from build123d import *

# Parameters (mm, degrees)
BOSS_EXTRUDE1_DEPTH = 5
SKETCH8_R           = 3.5
BOSS_EXTRUDE5_DEPTH = 1.5
SKETCH10_R          = 8
BOSS_EXTRUDE7_DEPTH = 5.75
SKETCH15_R          = 2.8
CUT_EXTRUDE7_DEPTH  = 10
NUT_CUT_START       = -1.5
SKETCH6_W           = 8.4
SKETCH6_H           = 8.4
NUT_CUT_DEPTH       = 46.182751545
SKETCH16_W          = 12
SKETCH16_H          = 3
CUT_EXTRUDE8_DEPTH  = 23
SKETCH17_R          = 2.35
CUT_EXTRUDE9_DEPTH  = 28
CUT_EXTRUDE10_START = 1.5
SKETCH19_R          = 6.25
CUT_EXTRUDE10_DEPTH = 46.182751545
CUT_EXTRUDE11_START = -8
CUT_EXTRUDE11_DEPTH = 3.8
LPATTERN1_COUNT     = 2
LPATTERN1_PITCH     = 10
SKETCH22_R          = 3.051848234
BOSS_EXTRUDE8_DEPTH = 0.65
SKETCH23_R          = 3.919040969
BOSS_EXTRUDE9_DEPTH = 0.65


with BuildPart() as part:
    # Sketch1 → Boss-Extrude1 (new body)
    with BuildSketch(Plane.XY):
        with BuildLine():
            Line((-40.155138696, -0.836255417), (-17.155138696, -0.836255417))
            Line((-17.155138696, -0.836255417), (-5.68921993, -10.190248634))
            ThreePointArc((-5.68921993, -10.190248634), (6.973720426, -8.905748138), (5.68921993, 3.757192218))
            Line((5.68921993, 3.757192218), (-10.744236538, 17.163744583))
            Line((-10.744236538, 17.163744583), (-40.155138696, 17.163744583))
            Line((-40.155138696, 17.163744583), (-40.155138696, -0.836255417))
        make_face()
    extrude(amount=BOSS_EXTRUDE1_DEPTH)

    # Sketch8 → Boss-Extrude5 (add)
    with BuildSketch(Plane.XY.offset(5)):
        with Locations((0, -3.216528208)):
            Circle(SKETCH8_R)
    extrude(amount=BOSS_EXTRUDE5_DEPTH)

    # Sketch10 → section 0 of loft4
    with BuildSketch(Plane.XY.offset(5), mode=Mode.PRIVATE) as loft4_s0:
        with Locations((0, -3.216528208)):
            Circle(SKETCH10_R)
    # loft up to a face of the part (loft4)
    loft([loft4_s0.sketch, part.faces().sort_by_distance((0, -3.216528208, 6.5))[0]])

    # Sketch14 → Boss-Extrude7 (add)
    with BuildSketch(Plane.XY.offset(5)):
        with BuildLine():
            Line((-40.155138696, -0.836255417), (-40.155138696, 17.163744583))
            Line((-40.155138696, 17.163744583), (-10.744236538, 17.163744583))
            Line((-10.744236538, 17.163744583), (0.78858875, 7.75516846))
            ThreePointArc((0.78858875, 7.75516846), (-8.523436076, 3.736962818), (-10.589851111, -6.192272392))
            Line((-10.589851111, -6.192272392), (-17.155138696, -0.836255417))
            Line((-17.155138696, -0.836255417), (-40.155138696, -0.836255417))
        make_face()
    extrude(amount=BOSS_EXTRUDE7_DEPTH)

    # Sketch15 → Cut-Extrude7 (cut)
    with BuildSketch(Plane(origin=(0, 0, 0), x_dir=(-1, 0, 0), z_dir=(0, 0, -1))):
        with Locations((0, -3.216528208)):
            Circle(SKETCH15_R)
    extrude(amount=-CUT_EXTRUDE7_DEPTH, mode=Mode.SUBTRACT)

    # Mirror1: part across plane


with BuildPart() as part_1:
    add(part.part)
    add(part.part.mirror(Plane(origin=(0, -3.216528208, 10.75), x_dir=(1, 0, 0), z_dir=(0, 0, 1))))

    # Sketch6 → nut-cut (cut, through all)
    with BuildSketch(Plane.XY.offset(5).offset(NUT_CUT_START)):
        with Locations((0, -3.216528208)):
            Rectangle(SKETCH6_W, SKETCH6_H)
    extrude(amount=-NUT_CUT_DEPTH, mode=Mode.SUBTRACT)

    # Sketch16 → Cut-Extrude8 (cut)
    with BuildSketch(Plane.ZY.offset(40.155138696)):
        with Locations((10.75, 0.663744583)):
            Rectangle(SKETCH16_W, SKETCH16_H)
        with Locations((10.75, 15.663744583)):
            Rectangle(SKETCH16_W, SKETCH16_H)
    extrude(amount=-CUT_EXTRUDE8_DEPTH, mode=Mode.SUBTRACT)

    # Sketch17 → Cut-Extrude9 (cut)
    with BuildSketch(Plane.ZY.offset(40.155138696)):
        with Locations((10.75, 8.163744583)):
            Circle(SKETCH17_R)
    extrude(amount=-CUT_EXTRUDE9_DEPTH, mode=Mode.SUBTRACT)

    # Sketch19 → Cut-Extrude10 (cut, through all)
    with BuildSketch(Plane.XY.offset(16.5).offset(CUT_EXTRUDE10_START)):
        with Locations(Location((0, -3.216528208, 0), (0, 0, 180))):
            Circle(SKETCH19_R)
    extrude(amount=CUT_EXTRUDE10_DEPTH, mode=Mode.SUBTRACT)

    # Sketch20 → Cut-Extrude11 (cut)
    with BuildSketch(Plane.ZY.offset(40.155138696).offset(CUT_EXTRUDE11_START)):
        Polygon((7, 14.163744583), (14.5, 14.163744583), (14.5, 5.998681073), (10.75, 3.833617564), (7, 5.998681073), align=None)
    cut_extrude11 = extrude(amount=-CUT_EXTRUDE11_DEPTH, mode=Mode.SUBTRACT)

    # LPattern1: Cut-Extrude11 ×2
    with Locations(*[(i * LPATTERN1_PITCH, 0, 0) for i in range(1, LPATTERN1_COUNT)]):
        add(cut_extrude11, mode=Mode.SUBTRACT)

    # Sketch22 → Boss-Extrude8 (add)
    with BuildSketch(Plane(origin=(0, 0, 6.5), x_dir=(-1, 0, 0), z_dir=(0, 0, -1))):
        with Locations((0, -3.216528208)):
            Circle(SKETCH22_R)
    extrude(amount=BOSS_EXTRUDE8_DEPTH)

    # Sketch23 → Boss-Extrude9 (add)
    with BuildSketch(Plane.XY.offset(18)):
        with Locations((0, -3.216528208)):
            Circle(SKETCH23_R)
    extrude(amount=-BOSS_EXTRUDE9_DEPTH)


solid = part_1.part
Read the model definition and answer for the solid it produces. Units are mm, in the model's axes. A direction names the side the tool comes from. Round coordinates to 2 decimals unless told otherwise and drop trailing zeros. Order: outer loops, then holes, each group sorted by start corner. A loop starts at its lowest first (then second) coordinate and runs counter-clockwise, first axis right, second up.
1) Straight lines are drawn through the part: L1, parallel to Z at x = -18, y = 0.5; L2, parallel to Z at x = -8.5, y = -5.75; L3, parallel to X at y = 12.75, z = 7.5. For each, find the intervals that lie inside material, in ascending order.
2) The part is cut by section A-A on x = -30. Write down the section's boundary in (y, z), plus the area to 3 significant figures.
3) The mould has two halves that part along X. Classify faces 1 (the face through (-0.806, -6.847, 6.427)), 2 (the face through (-29, 1, 16.75)), 3 (the face through (-17.155, 1, 11)): released by +X, released by -X, zero draft, split by the parting line, or undercut.
4) The part is cut by section C-C on x = -23.5. Write down the section's boundary in (y, z).
5) The part is cut by section D-D on z = 20. Write down the section's boundary in (x, y), plus the area to 3 significant figures.
6) For faces 4 (the face through (-36.21, 6.73, 8.89)), 5 (the face through (-1.29, -5.7, 16.19)), 6 (the face through (-2, -1, 15)), determine the directions among +Z, -Z, +X, -X, +Y, -Y from which every point of the face is accessible in a straight line to the end or side of a thin tool.
7) The part is cut by section B-B on z = 3. Write down the section's boundary in (x, y), plus the area to 3 significant figures.
8) Flat-ended cylindrical pins translate along their axes: pin 1 (4.5 mm diameter, centred on x = 0, y = -3.22, fed in from -Z); pin 2 (2.5 mm diameter, centred on y = 8.5, z = 11.5, fed in from -X); pin 3 (2 mm diameter, centred on y = 5, z = 8.5, fed in from +X). Find the tip coordinate at first contact, or state that the pin passes through.
Resolved:
1. L1: z = 0 to 4.75, 16.75 to 21.5
1. L2: z = 0 to 5, 16.5 to 21.5
1. L3: x = -40.16 to -32.16, -28.36 to -22.16, -18.36 to -5.33
2. outline: (-0.84, 0) - (17.16, 0) - (17.16, 4.75) - (14.16, 4.75) - (14.16, 7) - (6, 7) - (3.83, 10.75) - (6, 14.5) - (14.16, 14.5) - (14.16, 16.75) - (17.16, 16.75) - (17.16, 21.5) - (-0.84, 21.5) - (-0.84, 16.75) - (2.16, 16.75) - (2.16, 4.75) - (-0.84, 4.75) - close
2. area: 246 mm2
3. face 1: undercut
3. face 2: zero draft
3. face 3: released by -X
4. outline: (-0.84, 0) - (17.16, 0) - (17.16, 4.75) - (14.16, 4.75) - (14.16, 16.75) - (17.16, 16.75) - (17.16, 21.5) - (-0.84, 21.5) - (-0.84, 16.75) - (2.16, 16.75) - (2.16, 4.75) - (-0.84, 4.75) - close; hole circle Ø4.7 at (8.16, 10.75)
5. outline: (-40.16, -0.84) - (-17.16, -0.84) - (-5.69, -10.19) arc R9 ccw to (5.69, 3.76) - (-10.74, 17.16) - (-40.16, 17.16) - close; hole circle Ø12.5 at (0, -3.22)
5. area: 800 mm2
6. face 4: -X
6. face 5: none
6. face 6: +X, -Y
7. outline: (-40.16, -0.84) - (-17.16, -0.84) - (-5.69, -10.19) arc R9 ccw to (5.69, 3.76) - (-10.74, 17.16) - (-40.16, 17.16) - close; hole (-4.2, -7.42) - (4.2, -7.42) - (4.2, 0.98) - (-4.2, 0.98) - close
7. area: 852 mm2
8. pin 1: stops at z = 5.85
8. pin 2: stops at x = -12.16
8. pin 3: stops at x = -6
